Autodesk Inventor part; units mm, degrees
ref_plane "YZ Plane" through (0, 0, 0) normal (1, 0, 0) x (0, 1, 0)
ref_plane "XZ Plane" through (0, 0, 0) normal (0, 1, 0) x (-1, 0, 0)
ref_plane "XY Plane" through (0, 0, 0) normal (0, 0, 1) x (1, 0, 0)
sketch "Sketch1" plane through (0, 0, 0) normal (0, 1, 0) x (-1, 0, 0)
  arc A0 (-5.3837, -3.1747) -> (-5.3833, 3.1753) centre (0, 0) ccw
  line L0 (-5.3833, 3.1753) -> (-7.8217, 3.1753)
  line L1 (-5.3837, -3.1747) -> (-7.8217, -3.1747)
  line L2 (-7.8217, 3.1753) -> (-7.8217, -3.1747)
  circle A1 centre (0, 0) radius 27.5 construction
  circle A2 centre (0, 0) radius 38
  arc A3 (37.5726, 5.6835) -> (34.9367, -14.9474) centre (37.6936, -4.8158) ccw
  arc A4 (27.0562, 26.6827) -> (37.0503, 8.4426) centre (33.3254, 18.2597) ccw
  arc A5 (6.2052, 37.4899) -> (25.0119, 28.6078) centre (16.228, 34.3606) ccw
  arc A6 (-17.0159, 33.9773) -> (3.4198, 37.8458) centre (-7.0679, 37.3369) ccw
  arc A7 (-33.7375, 17.4865) -> (-19.4786, 32.628) centre (-27.6641, 26.0518) ccw
  arc A8 (-37.5726, -5.6835) -> (-34.9367, 14.9474) centre (-37.6936, 4.8158) ccw
  arc A9 (-27.0562, -26.6827) -> (-37.0503, -8.4426) centre (-33.3254, -18.2597) ccw
  arc A10 (-6.2052, -37.4899) -> (-25.0119, -28.6078) centre (-16.228, -34.3606) ccw
  arc A11 (17.0159, -33.9773) -> (-3.4198, -37.8458) centre (7.0679, -37.3369) ccw
  arc A12 (33.7375, -17.4865) -> (19.4786, -32.628) centre (27.6641, -26.0518) ccw
  dimension "d0" = 12.5
  dimension "d1" = 6.35
  dimension "d2" = 2.4384
  dimension "d3" = 2.438
  dimension "d4" = 55
  dimension "d5" = 76
  dimension "d6" = 10.5
  dimension "d9" = 360
extrude "Extrusion1" add sketch "Sketch1" along normal blind 10 contours A3 A2 A12 A11 A10 A9 A8 A7 A6 A5 A4 | A4 A2 | A2 A12 | A5 A2 | A2 A11 | A6 A2 | A2 A10 | A7 A2 | A2 A9 | A8 A2
sketch "Sketch2" plane through (0, 10, 0) normal (0, 1, 0) x (1, 0, 0)
  arc A0 (-37.5726, -5.6835) -> (-34.9367, 14.9474) centre (-37.6936, 4.8158) ccw
  arc A1 (-37.5726, -5.6835) -> (-34.9367, 14.9474) centre (-37.6936, 4.8158) ccw
  circle A2 centre (0, 0) radius 38
  arc A3 (-27.0562, -26.6827) -> (-37.0503, -8.4426) centre (-33.3254, -18.2597) ccw
hole "Hole1" at (-33.3254, 10, 18.2597) direction (0, -1, 0) diameter 21 end through all
pattern_circular "Circular Pattern1" count 10 over 360 about axis through (0, 10, 0) along (0, -1, 0) of "Hole1"
properties part number "gear"
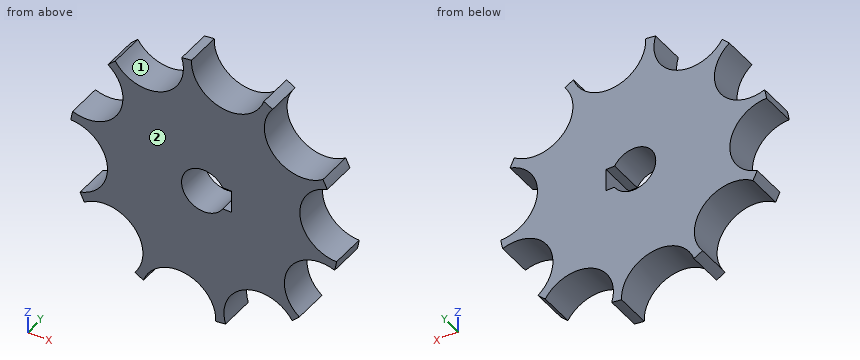
Work out the finished part from the listing and answer in its coordinate system (mm). Face numbers are marked on the shaded views. Give positions to 0.01 mm unless a question says otherwise; leave off trailing zeros. Write each loop counter-clockwise with the first axis right and the second up, starting at its lowest first coordinate (ties: lowest second). Pieces come first, ordered by that corner, then holes.
(1) The part is cut by section A-A on x = 1. Write down the section's boundary in (y, z), plus the area to 3 significant figures.
Final values:
outline: (0, -30.62) - (10, -30.62) - (10, -6.17) - (0, -6.17) - close; (0, 6.17) - (10, 6.17) - (10, 28.77) - (0, 28.77) - close
area: 470 mm2
(2) Straight lines are drawn through the part: line 1 (X direction, y = 1.5, z = 31.5); line 2 (Z direction, x = 34, y = 8.25); line 3 (X direction, y = 8, z = -1.5). For each, find the intervals that lie inside material, in ascending order.
Final values:
line 1: x = -6.13 to -1.66, 15.8 to 18.69
line 2: z = -7.78 to -5.01, 14.64 to 16.97
line 3: x = -27.73 to -6.07, 7.82 to 29.31
(3) The part is cut by section C-C on y = 4.75. Write down the section's boundary in (x, z).
Final values:
outline: (-37.57, 5.68) arc R10.5 cw to (-34.94, -14.95) arc R38 ccw to (-33.74, -17.49) arc R10.5 cw to (-19.48, -32.63) arc R38 ccw to (-17.02, -33.98) arc R10.5 cw to (3.42, -37.85) arc R38 ccw to (6.21, -37.49) arc R10.5 cw to (25.01, -28.61) arc R38 ccw to (27.06, -26.68) arc R10.5 cw to (37.05, -8.44) arc R38 ccw to (37.57, -5.68) arc R10.5 cw to (34.94, 14.95) arc R38 ccw to (33.74, 17.49) arc R10.5 cw to (19.48, 32.63) arc R38 ccw to (17.02, 33.98) arc R10.5 cw to (-3.42, 37.85) arc R38 ccw to (-6.21, 37.49) arc R10.5 cw to (-25.01, 28.61) arc R38 ccw to (-27.06, 26.68) arc R10.5 cw to (-37.05, 8.44) arc R38 ccw to start; hole (5.38, -3.17) - (7.82, -3.17) - (7.82, 3.18) - (5.38, 3.18) arc R6.25 ccw (long way) to start
(4) Flat-ended cylindrical pins translate along their axes: pin 1 Ø4 at (x, y) = (-12, 8.5) entering from +Z; pin 2 Ø5 at (y, z) = (2.5, 0) entering from -X; pin 3 Ø2 at (x, y) = (6.5, 5) entering from +Z; pin 4 Ø10 at (x, z) = (0, 0) entering from -Y. Find the tip coordinate at first contact, or state that the pin passes through.
Final values:
pin 1: stops at z = 25.91
pin 2: stops at x = -30.16
pin 3: stops at z = 26.95
pin 4: passes through
(5) The part is cut by section B-B on z = 25. Write down the section's boundary in (x, y), plus the area to 3 significant figures.
Final values:
outline: (-25.27, 0) - (-20.99, 0) - (-20.99, 10) - (-25.27, 10) - close; (-11.47, 0) - (17.22, 0) - (17.22, 10) - (-11.47, 10) - close
area: 330 mm2
(6) The part is cut by section D-D on x = -12. Write down the section's boundary in (y, z).
Final values:
outline: (0, -28.07) - (10, -28.07) - (10, 24.75) - (0, 24.75) - close
(7) The mould has two halves that part along Z. Classify the marked faces 1 and 2: pulls with the +Z half, pulls with the -Z half, needs draft (parallel to the pull), parting line crosses it, or undercut.
Final values:
face 1: undercut
face 2: needs draft
